The model under review builds one solid part; all positions refer to its coordinate system, in mm. Face numbers are marked on the shaded views. Round coordinates to 2 decimals unless told otherwise and drop trailing zeros. Order: outer loops, then holes, each group sorted by start corner. A loop starts at its lowest first (then second) coordinate and runs counter-clockwise, first axis right, second up.
```python
from build123d import *

# Parameters (mm, degrees)
SKETCH_1_R          = 41.5
SKETCH_1_R_2        = 29
EXTRUDE_1_DEPTH     = 33
SKETCH_2_R          = 41.5
EXTRUDE_2_DEPTH     = 3
SKETCH_3_R          = 2
CUT_EXTRUDE_1_DEPTH = 4
SKETCH_4_R          = 5.5
SKETCH_4_R_2        = 3
EXTRUDE_3_DEPTH     = 35


with BuildPart() as part:
    # 草图1 → 凸台-拉伸1 (new body)
    with BuildSketch(Plane(origin=(0, 0, 0), x_dir=(1, 0, 0), z_dir=(0, 1, 0))):
        Circle(SKETCH_1_R)
        Circle(SKETCH_1_R_2, mode=Mode.SUBTRACT)
    extrude(amount=EXTRUDE_1_DEPTH)

    # 草图2 → 凸台-拉伸2 (add)
    with BuildSketch(Plane.XZ):
        Circle(SKETCH_2_R)
    extrude(amount=EXTRUDE_2_DEPTH)

    # 草图3 → 切除-拉伸1 (cut, through all)
    with BuildSketch(Plane(origin=(0, 0, 0), x_dir=(1, 0, 0), z_dir=(0, 1, 0))):
        Circle(SKETCH_3_R)
    extrude(amount=-CUT_EXTRUDE_1_DEPTH, mode=Mode.SUBTRACT)

    # 草图4 → 凸台-拉伸3 (add)
    with BuildSketch(Plane(origin=(0, 0, 0), x_dir=(1, 0, 0), z_dir=(0, 1, 0))):
        Circle(SKETCH_4_R)
        Circle(SKETCH_4_R_2, mode=Mode.SUBTRACT)
    extrude(amount=EXTRUDE_3_DEPTH)


solid = part.part
```
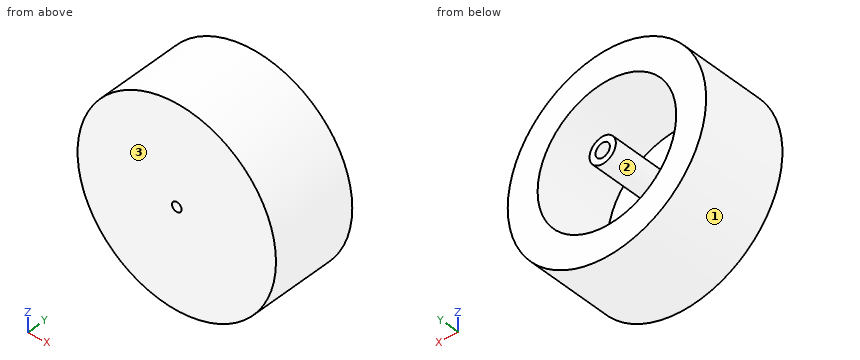
(1) Consider section A-A (x = 0). Write out the cut boundary in (y, z), and give its area (3 significant figures).
Data:
outline: (-3, -41.5) - (33, -41.5) - (33, -29) - (0, -29) - (0, -5.5) - (35, -5.5) - (35, -3) - (0, -3) - (0, -2) - (-3, -2) - close; (-3, 2) - (0, 2) - (0, 3) - (35, 3) - (35, 5.5) - (0, 5.5) - (0, 29) - (33, 29) - (33, 41.5) - (-3, 41.5) - close
area: 1,240 mm2
(2) Consider section D-D (x = -15.5). Write out the cut boundary in (y, z).
Data:
outline: (-3, -38.5) - (33, -38.5) - (33, -24.51) - (0, -24.51) - (0, 24.51) - (33, 24.51) - (33, 38.5) - (-3, 38.5) - close
(3) To check wall thickness, follow probe 1 along X at (y, z) = (27, 0); probe 2 along Z at (x, y) = (0, -2.3). State the ranges of each line that lie inside material, in increasing order.
Data:
probe 1: x = -41.5 to -29, -5.5 to -3, 3 to 5.5, 29 to 41.5
probe 2: z = -41.5 to -2, 2 to 41.5
(4) Insertion check: pin 1 (4.5 mm diameter, centred on x = 0, z = 0, fed in from +Y); pin 2 (3 mm diameter, centred on x = -6, y = 14.5, fed in from +Z); pin 3 (8 mm diameter, centred on y = 5.5, z = 6, fed in from -X); pin 4 (1 mm diameter, centred on x = 0.5, z = 0.5, fed in from +Y). Each pin has a flat end and moves straight along its axis. Give the tip position at first contact, or say it passes through.
Data:
pin 1: stops at y = 0
pin 2: stops at z = 41.26
pin 3: stops at x = -41.45
pin 4: passes through
(5) Draft analysis for pull direction Z (two halves, no side actions). For the marked faces 1, 2 and 3, state which applies: pulls with the +Z half, pulls with the -Z half, needs draft (parallel to the pull), parting line crosses it, or undercut.
Data:
face 1: parting line crosses it
face 2: undercut
face 3: needs draft
(6) Consider section B-B (z = 0). Write out the cut boundary in (x, y), and give its area (3 significant figures).
Data:
outline: (-41.5, -3) - (-2, -3) - (-2, 0) - (-3, 0) - (-3, 35) - (-5.5, 35) - (-5.5, 0) - (-29, 0) - (-29, 33) - (-41.5, 33) - close; (2, -3) - (41.5, -3) - (41.5, 33) - (29, 33) - (29, 0) - (5.5, 0) - (5.5, 35) - (3, 35) - (3, 0) - (2, 0) - close
area: 1,240 mm2
(7) Consider section C-C (y = 15). Write out the cut boundary in (x, z), and give its area (3 significant figures).
Data:
outline: circle Ø83 at (0, 0); circle Ø11 at (0, 0); hole circle Ø58 at (0, 0); hole circle Ø6 at (0, 0)
area: 2,840 mm2
